Work out the finished part from the listing and answer in its coordinate system (mm). A direction names the side the tool comes from. Coordinates: 2 decimals unless noted, no trailing zeros. Write each loop counter-clockwise with the first axis right and the second up, starting at its lowest first coordinate (ties: lowest second). Pieces come first, ordered by that corner, then holes. Notation, with made-up numbers: M 84.5,50 L 137.5,50 A8 ccw 137.5,58 Z; hole C 50.25,67 d1. An arc over 180 degrees is marked long. Use CSV: the item, a comma, the result in double quotes.
Autodesk Inventor part; units mm, degrees
ref_plane "YZ Plane" through (0, 0, 0) normal (1, 0, 0) x (0, 1, 0)
ref_plane "XZ Plane" through (0, 0, 0) normal (0, 1, 0) x (-1, 0, 0)
ref_plane "XY Plane" through (0, 0, 0) normal (0, 0, 1) x (1, 0, 0)
sketch "Sketch1" plane through (0, 0, 0) normal (0, 1, 0) x (-1, 0, 0)
  circle A0 centre (0, 0) radius 8
  dimension "d0" = 16
extrude "Extrusion1" add sketch "Sketch1" along normal blind 32
sketch "Sketch2" plane through (0, 32, 0) normal (0, 1, 0) x (1, 0, 0)
  circle A0 centre (0, 0) radius 8
  circle A1 centre (0, 0) radius 3
  point P0 (5.5, 0)
  point P1 (-5.5, 0)
  dimension "d3" = 6
  dimension "d4" = 5.5
  dimension "d7" = 360
extrude "Extrusion2" add sketch "Sketch2" along normal blind 1.5 contours A1
hole "Hole1" at (5.5, 32, 0) at (-5.5, 32, 0) direction (0, -1, 0) diameter 1.567 depth 3 tip angle 118
sketch "Sketch3" plane through (0, 33.5, 0) normal (0, 1, 0) x (1, 0, 0)
  circle A0 centre (0, 0) radius 3
  circle A1 centre (0, 0) radius 2
  dimension "d18" = 4
extrude "Extrusion3" add sketch "Sketch3" along normal blind 10 contours A1
sketch "Sketch4" plane through (0, 43.5, 0) normal (0, 1, 0) x (1, 0, 0)
  circle A0 centre (0, 0) radius 2
  arc A1 (1.7321, 1) -> (-1.7321, 1) centre (0, 0) ccw
  line L0 (-1.7321, 1) -> (1.7321, 1)
  dimension "d21" = 1
  dimension "d23" = 1
extrude "Extrusion4" cut sketch "Sketch4" against normal blind 7.5 contours L0 A0 picked at (0.4849, 1.1242)
sketch "Sketch5" plane through (0, 0, 0) normal (0, -1, 0) x (1, 0, 0)
  circle A0 centre (0, 0) radius 8
  circle A1 centre (0, 0) radius 2.5
  dimension "d26" = 5
extrude "Extrusion5" add sketch "Sketch5" along normal blind 1 contours A1
properties part number "motor_43dsd"
Item 1: Consider probe 1 along Y at (x, z) = (-5.5, -4.75); probe 2 along Z at (x, y) = (5.5, 30.7); probe 3 along X at (y, z) = (31, -0.5). Determine where each line is inside the solid, lowest interval first.
Answer:
probe 1,"y = 0 to 32"
probe 2,"z = -5.81 to -0.78, 0.78 to 5.81"
probe 3,"x = -7.98 to -6.1, -4.9 to 4.9, 6.1 to 7.98"
Item 2: The part is cut by section C-C (y = 30.5). Write down the section's boundary in (x, z).
Answer:
outline,"C 0,0 d16; hole C -5.5,0 d1.57; hole C 5.5,0 d1.57"
Item 3: The part is cut by section D-D (z = 7). Write down the section's boundary in (x, y), then the cut area to 3 significant figures.
Answer:
outline,"M -3.87,0 L 3.87,0 L 3.87,32 L -3.87,32 Z"
area,"248 mm2"
Item 4: For a pull along X with two mould halves and no side action, classify faces 5 (the face through (-3, 33, 0)), 6 (the face through (-3.4, 32, 0.1)), 7 (the face through (-6.277, 30.479, -0.102)) as released by +X, released by -X, zero draft, split by the parting line, or undercut.
Answer:
face 5,"split by the parting line"
face 6,"zero draft"
face 7,"undercut"
Item 5: The part is cut by section B-B (y = 3). Write down the section's boundary in (x, z), then the cut area to 3 significant figures.
Answer:
outline,"C 0,0 d16"
area,"201 mm2"
Item 6: A tool of negligible diameter and unlimited length cuts with its end or side. For faces 1 (the face through (-0.54, -0.49, 2.44)), 2 (the face through (0, 36, -1.4)), 3 (the face through (1.73, 15.78, 7.81)), 4 (the face through (4.723, 30.479, -0.102)), from which of +Z, -Z, +X, -X, +Y, -Y can it reach the whole face along a straight path? Write none if from no direction.
Answer:
face 1,"-Y"
face 2,"-Z, +X, -X, +Y"
face 3,"+Y, -Y"
face 4,"+Y"
Item 7: Given pin 1 (2 mm diameter, centred on x = 3, z = 4, fed in from +Y); pin 2 (2 mm diameter, centred on x = -5.5, y = 28, fed in from +Z); pin 3 (8 mm diameter, centred on y = 10.5, z = -5.5, fed in from -X), each flat-ended and moving along its own axis, determine where each tip first touches the part or whether it passes through.
Answer:
pin 1,"stops at y = 32"
pin 2,"stops at z = 6.61"
pin 3,"stops at x = -7.86"
Item 8: The part is cut by section A-A (x = 0). Write down the section's boundary in (y, z).
Answer:
outline,"M -1,-2.5 L 0,-2.5 L 0,-8 L 32,-8 L 32,-3 L 33.5,-3 L 33.5,-2 L 36,-2 L 36,-1 L 43.5,-1 L 43.5,2 L 33.5,2 L 33.5,3 L 32,3 L 32,8 L 0,8 L 0,2.5 L -1,2.5 Z"
